Can you work these out from the model? Positions are in its coordinate system, mm. A direction names the side the tool comes from. Give positions to 0.01 mm unless a question says otherwise; leave off trailing zeros. Order: outer loops, then holes, each group sorted by start corner. A loop starts at its lowest first (then second) coordinate and runs counter-clockwise, first axis right, second up. Notation, with made-up numbers: (65, 36) - (83, 36) arc R17 cw to (83, 62) - close; hole circle Ø6 at (53.25, 21.25). An arc over 180 degrees is marked (long way). One line per question, with ' | ' between items.
```python
from build123d import *

# Parameters (mm, degrees)
BOSS_EXTRUDE1_DEPTH = 10
SKETCH2_R           = 25
SKETCH2_R_2         = 16
BOSS_EXTRUDE2_DEPTH = 35
BOSS_EXTRUDE4_START = -45
BOSS_EXTRUDE4_DEPTH = 35
SKETCH4_R           = 5
CUT_EXTRUDE1_DEPTH  = 35
FILLET1_R           = 12
FILLET2_R           = 12
BOSS_EXTRUDE5_START = -5
SKETCH5_R           = 19
SKETCH5_R_2         = 10
BOSS_EXTRUDE5_DEPTH = 8
BOSS_EXTRUDE6_DEPTH = 10
FILLET3_R           = 6
FILLET4_START       = 35
FILLET4_DEPTH       = 10
FILLET4_START_2     = -78
FILLET4_2_DEPTH     = 21.60438079
FILLET4_START_3     = 30.318225383
FILLET4_3_DEPTH     = 4.681774617
BOSS_EXTRUDE7_START = -5
SKETCH7_R           = 10
BOSS_EXTRUDE7_DEPTH = 8
BOSS_EXTRUDE8_START = -10
BOSS_EXTRUDE8_DEPTH = 10
FILLET5_R           = 6


with BuildPart() as part:
    # Sketch1 → Boss-Extrude1 (new body)
    with BuildSketch(Plane(origin=(0, 0, 0), x_dir=(1, 0, 0), z_dir=(0, 1, 0))):
        with BuildLine():
            Line((-45, 0), (45, 0))
            Line((45, 0), (45, 40))
            Line((45, 40), (69, 40))
            Line((69, 40), (69, 72))
            ThreePointArc((69, 72), (70.757359313, 76.242640687), (75, 78))
            Line((75, 78), (-75, 78))
            ThreePointArc((-75, 78), (-70.757359313, 76.242640687), (-69, 72))
            Line((-69, 72), (-69, 40))
            Line((-69, 40), (-45, 40))
            Line((-45, 40), (-45, 0))
        make_face()
    extrude(amount=-BOSS_EXTRUDE1_DEPTH)

    # Sketch2 → Boss-Extrude2 (add)
    with BuildSketch(Plane(origin=(0, 0, 0), x_dir=(1, 0, 0), z_dir=(0, 1, 0))):
        with Locations(Location((0, 28, 0), (0, 0, 270))):
            Circle(SKETCH2_R)
        with Locations(Location((0, 28, 0), (0, 0, 270))):
            Circle(SKETCH2_R_2, mode=Mode.SUBTRACT)
    extrude(amount=BOSS_EXTRUDE2_DEPTH)

    # Sketch3 → Boss-Extrude4 (add)
    with BuildSketch(Plane(origin=(0, 35, 0), x_dir=(1, 0, 0), z_dir=(0, 1, 0)).offset(BOSS_EXTRUDE4_START)):
        with BuildLine():
            Line((32, 63), (-32, 63))
            ThreePointArc((-32, 63), (-34.121320344, 63.878679656), (-35, 66))
            Line((-35, 66), (-35, 88))
            Line((-35, 88), (-75, 88))
            Line((-75, 88), (-75, 78))
            Line((-75, 78), (-45, 78))
            Line((-45, 78), (-45, 65))
            ThreePointArc((-45, 65), (-41.485281374, 56.514718626), (-33, 53))
            Line((-33, 53), (-25, 53))
            Line((-25, 53), (-25, 28))
            ThreePointArc((-25, 28), (0, 53), (25, 28))
            Line((25, 28), (25, 53))
            Line((25, 53), (33, 53))
            ThreePointArc((33, 53), (41.485281374, 56.514718626), (45, 65))
            Line((45, 65), (45, 78))
            Line((45, 78), (75, 78))
            Line((75, 78), (75, 88))
            Line((75, 88), (35, 88))
            Line((35, 88), (35, 66))
            ThreePointArc((35, 66), (34.121320344, 63.878679656), (32, 63))
        make_face()
    extrude(amount=BOSS_EXTRUDE4_DEPTH)

    # Sketch4 → Cut-Extrude1 (cut)
    with BuildSketch(Plane.XY.offset(-78)):
        with Locations((63, 13)):
            Circle(SKETCH4_R)
    cut_extrude1 = extrude(amount=-CUT_EXTRUDE1_DEPTH, mode=Mode.SUBTRACT)

    # Mirror1: Cut-Extrude1 across plane
    add(cut_extrude1.mirror(Plane(origin=(0, 0, 0), x_dir=(0, 0, 1), z_dir=(1, 0, 0))), mode=Mode.SUBTRACT)

    # Fillet1
    fillet1_edges = [part.edges().sort_by_distance(p)[0] for p in [
        (-45, -5, -40),
        (45, -5, -40),
    ]]
    fillet(fillet1_edges, radius=FILLET1_R)

    # Fillet2
    fillet2_edges = [part.edges().sort_by_distance(p)[0] for p in [
        (-69, -5, -40),
        (69, -5, -40),
    ]]
    fillet(fillet2_edges, radius=FILLET2_R - 0.0001)  # a hair under: the kernel refuses the full size



with BuildPart() as body_2:
    # Sketch5 → Boss-Extrude5 (new, symmetric)
    with BuildSketch(Plane(origin=(45, 0, 0), x_dir=(0, 0, -1), z_dir=(1, 0, 0)).offset(BOSS_EXTRUDE5_START)):
        with Locations((28, -66)):
            Circle(SKETCH5_R)
        with Locations((28, -66)):
            Circle(SKETCH5_R_2, mode=Mode.SUBTRACT)
    extrude(amount=BOSS_EXTRUDE5_DEPTH, both=True)


with BuildPart() as part_1:
    add(part.part)

    add(body_2.part)  # Boss-Extrude6 merges body 2
    # Sketch5<3> → Boss-Extrude6 (add)
    with BuildSketch(Plane(origin=(45, 0, 0), x_dir=(0, 0, -1), z_dir=(1, 0, 0))):
        with BuildLine():
            Line((61, -10), (0, -10))
            Line((0, -10), (9.228717941, -68.939212458))
            ThreePointArc((9.228717941, -68.939212458), (26.525951004, -47.057265785), (47, -66))
            ThreePointArc((47, -66), (46.868026287, -68.235527685), (46.473938523, -70.439999487))
            Line((46.473938523, -70.439999487), (61, -10))
        make_face()
    extrude(amount=-BOSS_EXTRUDE6_DEPTH)

    # Fillet3
    fillet3_edges = [part_1.edges().sort_by_distance(p)[0] for p in [
        (35, -10, -30.5),
    ]]
    fillet(fillet3_edges, radius=FILLET3_R)

    # Fillet4: read off the stored shape, not the designer's step
    # Fillet4 outline → Fillet4 (add)
    with BuildSketch(Plane.YZ.offset(FILLET4_START)):
        with BuildLine():
            ThreePointArc((-29.157895412, -56.39561931), (-15.365176157, -65.228495591), (-10, -80.703433157))
            Line((-10, -80.703433157), (-10, -61))
            Line((-10, -61), (-29.157895412, -56.39561931))
        make_face()
    extrude(amount=FILLET4_DEPTH)

    # Fillet4 2 outline → Fillet4 2 (add)
    with BuildSketch(Plane.XY.offset(FILLET4_START_2)):
        with BuildLine():
            ThreePointArc((29, -10), (33.242640687, -11.757359313), (35, -16))
            Line((35, -16), (35, -10))
            Line((35, -10), (29, -10))
        make_face()
    extrude(amount=FILLET4_2_DEPTH)

    # Fillet4 3 outline → Fillet4 3 (cut)
    with BuildSketch(Plane.YZ.offset(FILLET4_START_3)):
        with BuildLine():
            Line((-18, -80), (-10.009898324, -80))
            ThreePointArc((-10.009898324, -80), (-12.047126523, -70.795577731), (-17.3481317, -63))
            Line((-17.3481317, -63), (-18, -63))
            Line((-18, -63), (-18, -80))
        make_face()
    extrude(amount=FILLET4_3_DEPTH, mode=Mode.SUBTRACT)



with BuildPart() as body_2_2:
    # Sketch7 → Boss-Extrude7 (new, symmetric)
    with BuildSketch(Plane.ZY.offset(45).offset(BOSS_EXTRUDE7_START)):
        with BuildLine():
            ThreePointArc((-46.473938523, -70.439999487), (-28, -85), (-9.526061477, -70.439999487))
            Line((-9.526061477, -70.439999487), (-9.055986357, -67.457514009))
            ThreePointArc((-9.055986357, -67.457514009), (-9.014001748, -66.729294447), (-9, -66))
            ThreePointArc((-9, -66), (-30.235527685, -47.131973713), (-46.473938523, -70.439999487))
        make_face()
        with Locations(Location((-28, -66, 0), (0, 0, 180))):
            Circle(SKETCH7_R, mode=Mode.SUBTRACT)
    extrude(amount=BOSS_EXTRUDE7_DEPTH, both=True)


with BuildPart() as part_2:
    add(part_1.part)

    add(body_2_2.part)  # Boss-Extrude8 merges body 2 2
    # Sketch7<3> → Boss-Extrude8 (add)
    with BuildSketch(Plane.ZY.offset(45).offset(BOSS_EXTRUDE8_START)):
        with BuildLine():
            ThreePointArc((-9, -66), (-9.014001748, -66.729294447), (-9.055986357, -67.457514009))
            Line((-9.055986357, -67.457514009), (0, -10))
            Line((0, -10), (-28, -10))
            Line((-28, -10), (-78, -10))
            Line((-78, -10), (-70.785998867, -12.051263714))
            Line((-70.785998867, -12.051263714), (-64.455356347, -16))
            Line((-64.455356347, -16), (-59.38495245, -21.941578182))
            Line((-59.38495245, -21.941578182), (-56.39561931, -29.157895412))
            Line((-56.39561931, -29.157895412), (-46.473938523, -70.439999487))
            ThreePointArc((-46.473938523, -70.439999487), (-30.235527685, -47.131973713), (-9, -66))
        make_face()
    extrude(amount=BOSS_EXTRUDE8_DEPTH)

    # Fillet5
    # the kernel refuses this fillet: 6 mm, written as the material it adds along each edge
    with BuildSketch(Plane(origin=(-35, -10, 0), x_dir=(1, 0, 0), z_dir=(0, 0, -1))) as fillet5_piece_1_section:
        with BuildLine():
            CenterArc((FILLET5_R, FILLET5_R), FILLET5_R, 180, 90)
            Line((0, FILLET5_R), (0, 0))
            Line((0, 0), (FILLET5_R, 0))
        make_face()
    fillet5_piece_1 = extrude(amount=78, mode=Mode.PRIVATE)
    fillet5_piece_1 = split(fillet5_piece_1, bisect_by=Plane(origin=(-35, -10, 0), z_dir=(0, 0.15568994877172856, -0.9878059727757555)), keep=Keep.TOP, mode=Mode.PRIVATE)
    fillet5_piece_1 = split(fillet5_piece_1, bisect_by=Plane(origin=(-35, -30.519826172, -5.834705883), z_dir=(0, 0.9618711340013946, 0.27350305587848817)), keep=Keep.TOP, mode=Mode.PRIVATE)
    fillet5_piece_1 = split(fillet5_piece_1, bisect_by=Plane(origin=(-35, -44.355068521, -40.257803859), z_dir=(0, 0.6491383227373216, 0.7606703871939389)), keep=Keep.TOP, mode=Mode.PRIVATE)
    add(fillet5_piece_1)
    with BuildSketch(Plane(origin=(-35, -10, 0), x_dir=(1, 0, 0), z_dir=(0, 0, -1))) as fillet5_piece_2_section:
        with BuildLine():
            CenterArc((FILLET5_R, FILLET5_R), FILLET5_R, 180, 90)
            Line((0, FILLET5_R), (0, 0))
            Line((0, 0), (FILLET5_R, 0))
        make_face()
    fillet5_piece_2 = extrude(amount=78, mode=Mode.PRIVATE)
    fillet5_piece_2 = split(fillet5_piece_2, bisect_by=Plane(origin=(-35, -30.519826172, -5.834705883), z_dir=(0, -0.9618711340013946, -0.27350305587848817)), keep=Keep.TOP, mode=Mode.PRIVATE)
    fillet5_piece_2 = split(fillet5_piece_2, bisect_by=Plane(origin=(-35, -44.355068521, -40.257803859), z_dir=(0, 0.6491383227373216, 0.7606703871939389)), keep=Keep.TOP, mode=Mode.PRIVATE)
    add(fillet5_piece_2)
    with BuildSketch(Plane(origin=(-35, -10, 0), x_dir=(1, 0, 0), z_dir=(0, 0, -1))) as fillet5_piece_3_section:
        with BuildLine():
            CenterArc((FILLET5_R, FILLET5_R), FILLET5_R, 180, 90)
            Line((0, FILLET5_R), (0, 0))
            Line((0, 0), (FILLET5_R, 0))
        make_face()
    fillet5_piece_3 = extrude(amount=78, mode=Mode.PRIVATE)
    fillet5_piece_3 = split(fillet5_piece_3, bisect_by=Plane(origin=(-35, -30.519826172, -5.834705883), z_dir=(0, 0.9618711340013946, 0.27350305587848817)), keep=Keep.TOP, mode=Mode.PRIVATE)
    fillet5_piece_3 = split(fillet5_piece_3, bisect_by=Plane(origin=(-35, -43.262700092, -20.747598748), z_dir=(0, 0.8484747516990396, 0.5292358602071983)), keep=Keep.TOP, mode=Mode.PRIVATE)
    fillet5_piece_3 = split(fillet5_piece_3, bisect_by=Plane(origin=(-35, -44.355068521, -40.257803859), z_dir=(0, -0.6491383227373216, -0.7606703871939389)), keep=Keep.TOP, mode=Mode.PRIVATE)
    add(fillet5_piece_3)
    with BuildSketch(Plane(origin=(-35, -10, 0), x_dir=(1, 0, 0), z_dir=(0, 0, -1))) as fillet5_piece_4_section:
        with BuildLine():
            CenterArc((FILLET5_R, FILLET5_R), FILLET5_R, 180, 90)
            Line((0, FILLET5_R), (0, 0))
            Line((0, 0), (FILLET5_R, 0))
        make_face()
    fillet5_piece_4 = extrude(amount=78, mode=Mode.PRIVATE)
    fillet5_piece_4 = split(fillet5_piece_4, bisect_by=Plane(origin=(-35, -30.519826172, -5.834705883), z_dir=(0, -0.9618711340013946, -0.27350305587848817)), keep=Keep.TOP, mode=Mode.PRIVATE)
    fillet5_piece_4 = split(fillet5_piece_4, bisect_by=Plane(origin=(-35, -43.262700092, -20.747598748), z_dir=(0, 0.8484747516990396, 0.5292358602071983)), keep=Keep.TOP, mode=Mode.PRIVATE)
    fillet5_piece_4 = split(fillet5_piece_4, bisect_by=Plane(origin=(-35, -44.355068521, -40.257803859), z_dir=(0, -0.6491383227373216, -0.7606703871939389)), keep=Keep.TOP, mode=Mode.PRIVATE)
    add(fillet5_piece_4)
    with BuildSketch(Plane(origin=(-35, -10, 0), x_dir=(1, 0, 0), z_dir=(0, 0, -1))) as fillet5_piece_5_section:
        with BuildLine():
            CenterArc((FILLET5_R, FILLET5_R), FILLET5_R, 180, 90)
            Line((0, FILLET5_R), (0, 0))
            Line((0, 0), (FILLET5_R, 0))
        make_face()
    fillet5_piece_5 = extrude(amount=78, mode=Mode.PRIVATE)
    fillet5_piece_5 = split(fillet5_piece_5, bisect_by=Plane(origin=(-35, -30.519826172, -5.834705883), z_dir=(0, 0.9618711340013946, 0.27350305587848817)), keep=Keep.TOP, mode=Mode.PRIVATE)
    fillet5_piece_5 = split(fillet5_piece_5, bisect_by=Plane(origin=(-35, -43.262700092, -20.747598748), z_dir=(0, -0.8484747516990396, -0.5292358602071983)), keep=Keep.TOP, mode=Mode.PRIVATE)
    add(fillet5_piece_5)


solid = part_2.part
```
(1) Will these pins go through, and if not, where does the flat tip stop? pin 1 (7.5 mm diameter, centred on x = 54, y = 15.5, fed in from +Z); pin 2 (16.5 mm diameter, centred on y = -55.5, z = -48, fed in from -X); pin 3 (12 mm diameter, centred on x = 54.5, y = -63.5, fed in from +Z); pin 4 (3 mm diameter, centred on x = -48.5, y = -58, fed in from +Z).
Answer below:
pin 1: z = -78 | pin 2: x = -48 | pin 3: through | pin 4: z = -10.18
(2) Imagine slicing it at A-A (y = 13). Count the separate pieces of the cut face and the enclosed holes in it, and give its area (3 significant figures).
Answer below:
separate pieces: 3 | enclosed holes: 1 | area: 3,170 mm^2
(3) Imagine slicing it at C-C (y = -19.5). List the corners of the cut face in (x, z) for me, and give its area (3 significant figures).
Answer below:
outline: (-45, -61.47) - (-35, -61.47) - (-35, -1.5) - (-45, -1.5) - close; (35, -61.09) - (45, -61.09) - (45, -1.49) - (35, -1.49) - close | area: 1,200 mm^2
(4) If we mould it in two halves opening along X, with no side actions, what happens to faces 6 (the face through (48, -74, -36)), 7 (the face through (-16.3, 35, -28.4)), 8 (the face through (0, 0, -71)), 9 (the face through (-45, -27, -31))? For each: released by +X, released by -X, zero draft, split by the parting line, or undercut.
Answer below:
face 6: released by +X | face 7: zero draft | face 8: undercut | face 9: released by -X
(5) If I drill on line 1 (Y direction, x = 35.5, z = -28); line 2 (X direction, y = -35, z = -51.5); line 3 (X direction, y = -57.5, z = -22.5), over which ranges is the centre line in solid material (lowest first)?
Answer below:
line 1: -85 to -76, -56 to 0 | line 2: -45 to -35, 35 to 45 | line 3: -48 to -32, 32 to 48
(6) Imagine slicing it at D-D (x = 27). List the corners of the cut face in (y, z) for me, and give its area (3 significant figures).
Answer below:
outline: (-10, -78) - (0, -78) - (0, -63) - (25, -63) - (25, -53) - (0, -53) - (0, 0) - (-10, 0) - close | area: 1,030 mm^2
(7) Imagine slicing it at B-B (x = -63). List the corners of the cut face in (y, z) for me.
Answer below:
outline: (-10, -88) - (8, -88) - (8, -78) - (0, -78) - (0, -41.61) - (-10, -41.61) - close; (18, -88) - (25, -88) - (25, -78) - (18, -78) - close
(8) On a 3-axis mill with a long thin cutter (end or side, diameter ignored), from which of +Z, -Z, +X, -X, +Y, -Y can I reach the whole of each face in a straight line? I mean faces 1 (the face through (70.711, -4.93, -76.196)), 2 (the face through (29, 12, -53)), 3 (the face through (-34, 0, -40)), 4 (the face through (40.112, -84.548, -23.881)), 5 (the face through (0, 12, -63)). Say none if no direction works.
Answer below:
face 1: +Z, +X, +Y, -Y | face 2: +Z, +X, +Y | face 3: +Z, +Y | face 4: none | face 5: -Z, +Y
